The model under review builds one solid part; all positions refer to its coordinate system, in mm. A direction names the side the tool comes from. Round coordinates to 2 decimals unless told otherwise and drop trailing zeros. Write each loop counter-clockwise with the first axis right and the second up, starting at its lowest first coordinate (ties: lowest second). Pieces come first, ordered by that corner, then holes. Notation, with made-up numbers: (35, -22.5) - (58, -22.5) arc R15 ccw to (58, -6.5) - close; hole circle Ø7 at (70, -38). An arc over 180 degrees is marked (long way). Return JSON: item names as keys, results as strings.
from build123d import *

# Parameters (mm, degrees)
SKETCH1_W               = 76.2
SKETCH1_H               = 228.6
BOSS_EXTRUDE1_DEPTH     = 38.1
SKETCH2_R               = 32.512
CUT_EXTRUDE2_DEPTH      = 244.959033446
SKETCH3_W               = 5.588
SKETCH3_H               = 15.705533419
BOSS_EXTRUDE2_DEPTH     = 228.6
SKETCH4_W               = 8.89
SKETCH4_H               = 5.08
CUT_EXTRUDE3_DEPTH      = 247.899646469
CRVPATTERN1_START       = -228.6
CRVPATTERN1_OUTLINE_W   = 5.588
CRVPATTERN1_OUTLINE_H   = 5.312766709
CRVPATTERN1_DEPTH       = 228.6
CRVPATTERN1_START_2     = -165.1
CRVPATTERN1_2_OUTLINE_W = 5.588
CRVPATTERN1_2_OUTLINE_H = 5.08
CRVPATTERN1_2_DEPTH     = 101.6
CRVPATTERN1_3_OUTLINE_W = 5.588
CRVPATTERN1_3_OUTLINE_H = 5.08
CRVPATTERN1_3_DEPTH     = 54.61
CRVPATTERN1_START_3     = -54.61
CRVPATTERN1_4_OUTLINE_W = 5.588
CRVPATTERN1_4_OUTLINE_H = 5.08
CRVPATTERN1_4_DEPTH     = 54.61
CRVPATTERN1_5_OUTLINE_W = 5.588
CRVPATTERN1_5_OUTLINE_H = 5.312766709
CRVPATTERN1_5_DEPTH     = 228.6
CRVPATTERN1_6_OUTLINE_W = 5.588
CRVPATTERN1_6_OUTLINE_H = 5.08
CRVPATTERN1_6_DEPTH     = 101.6
CRVPATTERN1_7_OUTLINE_W = 5.588
CRVPATTERN1_7_OUTLINE_H = 5.08
CRVPATTERN1_7_DEPTH     = 54.61
CRVPATTERN1_8_OUTLINE_W = 5.588
CRVPATTERN1_8_OUTLINE_H = 5.08
CRVPATTERN1_8_DEPTH     = 54.61
SKETCH6_W               = 215.9
SKETCH6_H               = 53.805533419
CUT_EXTRUDE4_DEPTH      = 328.736106382
CUT_EXTRUDE5_DEPTH      = 236.189892271
BOSS_EXTRUDE4_START     = -5.588
SKETCH8_W               = 35.618239262
SKETCH8_H               = 38.1
BOSS_EXTRUDE4_DEPTH     = 5.588
SKETCH9_R               = 4.191
CUT_EXTRUDE6_DEPTH      = 236.006490398


# Read off the part's stored shape, not the designer's step: CrvPattern1
with BuildPart() as part:
    # Sketch1 → Boss-Extrude1 (new body)
    with BuildSketch(Plane(origin=(0, 0, 0), x_dir=(1, 0, 0), z_dir=(0, 1, 0))):
        with Locations((38.1, 114.3)):
            Rectangle(SKETCH1_W, SKETCH1_H)
    extrude(amount=BOSS_EXTRUDE1_DEPTH)

    # Sketch2 → Cut-Extrude2 (cut, through all)
    with BuildSketch(Plane.XY):
        with Locations((38.1, 38.1)):
            Circle(SKETCH2_R)
    extrude(amount=-CUT_EXTRUDE2_DEPTH, mode=Mode.SUBTRACT)

    # Sketch3 → Boss-Extrude2 (add)
    with BuildSketch(Plane.XY):
        with Locations((2.794, 45.95276671)):
            Rectangle(SKETCH3_W, SKETCH3_H)
        with Locations((73.406, 45.95276671)):
            Rectangle(SKETCH3_W, SKETCH3_H)
    extrude(amount=-BOSS_EXTRUDE2_DEPTH)

    # Sketch4 → Cut-Extrude3 (cut, through all)
    with BuildSketch(Plane(origin=(76.2, 0, 0), x_dir=(0, 0, -1), z_dir=(1, 0, 0))):
        with Locations((59.055, 45.95276671)):
            Rectangle(SKETCH4_W, SKETCH4_H)
        with Locations((169.545, 45.95276671)):
            Rectangle(SKETCH4_W, SKETCH4_H)
    extrude(amount=-CUT_EXTRUDE3_DEPTH, mode=Mode.SUBTRACT)


with BuildPart() as body_2:
    # CrvPattern1 outline → CrvPattern1 (new body)
    with BuildSketch(Plane.XY.offset(CRVPATTERN1_START)):
        with BuildLine():
            Line((152.4, 43.41276671), (152.4, 0))
            Line((152.4, 0), (228.6, 0))
            Line((228.6, 0), (228.6, 43.41276671))
            Line((228.6, 43.41276671), (223.012, 43.41276671))
            Line((223.012, 43.41276671), (223.012, 38.1))
            ThreePointArc((223.012, 38.1), (190.5, 5.588), (157.988, 38.1))
            Line((157.988, 38.1), (157.988, 43.41276671))
            Line((157.988, 43.41276671), (152.4, 43.41276671))
        make_face()
        with Locations((155.194, 51.149150065)):
            Rectangle(CRVPATTERN1_OUTLINE_W, CRVPATTERN1_OUTLINE_H)
        with Locations((225.806, 51.149150065)):
            Rectangle(CRVPATTERN1_OUTLINE_W, CRVPATTERN1_OUTLINE_H)
    extrude(amount=CRVPATTERN1_DEPTH)

    # CrvPattern1 2 outline → CrvPattern1 2 (add)
    with BuildSketch(Plane.XY.offset(CRVPATTERN1_START_2)):
        with Locations((155.194, 45.95276671)):
            Rectangle(CRVPATTERN1_2_OUTLINE_W, CRVPATTERN1_2_OUTLINE_H)
        with Locations((225.806, 45.95276671)):
            Rectangle(CRVPATTERN1_2_OUTLINE_W, CRVPATTERN1_2_OUTLINE_H)
    extrude(amount=CRVPATTERN1_2_DEPTH)

    # CrvPattern1 3 outline → CrvPattern1 3 (add)
    with BuildSketch(Plane.XY.offset(CRVPATTERN1_START)):
        with Locations((155.194, 45.95276671)):
            Rectangle(CRVPATTERN1_3_OUTLINE_W, CRVPATTERN1_3_OUTLINE_H)
        with Locations((225.806, 45.95276671)):
            Rectangle(CRVPATTERN1_3_OUTLINE_W, CRVPATTERN1_3_OUTLINE_H)
    extrude(amount=CRVPATTERN1_3_DEPTH)

    # CrvPattern1 4 outline → CrvPattern1 4 (add)
    with BuildSketch(Plane.XY.offset(CRVPATTERN1_START_3)):
        with Locations((155.194, 45.95276671)):
            Rectangle(CRVPATTERN1_4_OUTLINE_W, CRVPATTERN1_4_OUTLINE_H)
        with Locations((225.806, 45.95276671)):
            Rectangle(CRVPATTERN1_4_OUTLINE_W, CRVPATTERN1_4_OUTLINE_H)
    extrude(amount=CRVPATTERN1_4_DEPTH)


with BuildPart() as body_3:
    # CrvPattern1 5 outline → CrvPattern1 5 (new body)
    with BuildSketch(Plane.XY.offset(CRVPATTERN1_START)):
        with BuildLine():
            Line((76.2, 43.41276671), (76.2, 0))
            Line((76.2, 0), (152.4, 0))
            Line((152.4, 0), (152.4, 43.41276671))
            Line((152.4, 43.41276671), (146.812, 43.41276671))
            Line((146.812, 43.41276671), (146.812, 38.1))
            ThreePointArc((146.812, 38.1), (114.3, 5.588), (81.788, 38.1))
            Line((81.788, 38.1), (81.788, 43.41276671))
            Line((81.788, 43.41276671), (76.2, 43.41276671))
        make_face()
        with Locations((78.994, 51.149150065)):
            Rectangle(CRVPATTERN1_5_OUTLINE_W, CRVPATTERN1_5_OUTLINE_H)
        with Locations((149.606, 51.149150065)):
            Rectangle(CRVPATTERN1_5_OUTLINE_W, CRVPATTERN1_5_OUTLINE_H)
    extrude(amount=CRVPATTERN1_5_DEPTH)

    # CrvPattern1 6 outline → CrvPattern1 6 (add)
    with BuildSketch(Plane.XY.offset(CRVPATTERN1_START_2)):
        with Locations((78.994, 45.95276671)):
            Rectangle(CRVPATTERN1_6_OUTLINE_W, CRVPATTERN1_6_OUTLINE_H)
        with Locations((149.606, 45.95276671)):
            Rectangle(CRVPATTERN1_6_OUTLINE_W, CRVPATTERN1_6_OUTLINE_H)
    extrude(amount=CRVPATTERN1_6_DEPTH)

    # CrvPattern1 7 outline → CrvPattern1 7 (add)
    with BuildSketch(Plane.XY.offset(CRVPATTERN1_START)):
        with Locations((78.994, 45.95276671)):
            Rectangle(CRVPATTERN1_7_OUTLINE_W, CRVPATTERN1_7_OUTLINE_H)
        with Locations((149.606, 45.95276671)):
            Rectangle(CRVPATTERN1_7_OUTLINE_W, CRVPATTERN1_7_OUTLINE_H)
    extrude(amount=CRVPATTERN1_7_DEPTH)

    # CrvPattern1 8 outline → CrvPattern1 8 (add)
    with BuildSketch(Plane.XY.offset(CRVPATTERN1_START_3)):
        with Locations((78.994, 45.95276671)):
            Rectangle(CRVPATTERN1_8_OUTLINE_W, CRVPATTERN1_8_OUTLINE_H)
        with Locations((149.606, 45.95276671)):
            Rectangle(CRVPATTERN1_8_OUTLINE_W, CRVPATTERN1_8_OUTLINE_H)
    extrude(amount=CRVPATTERN1_8_DEPTH)


with BuildPart() as cut_extrude4_tool:
    # Sketch6 → Cut-Extrude4 (new, through all)
    with BuildSketch(Plane.ZY):
        with Locations((-120.65, 26.90276671)):
            Rectangle(SKETCH6_W, SKETCH6_H)
    extrude(amount=-CUT_EXTRUDE4_DEPTH)


with BuildPart() as part_1:
    add(part.part)

    # Cut-Extrude4: cut by cut_extrude4_tool
    add(cut_extrude4_tool.part, mode=Mode.SUBTRACT)


with BuildPart() as body_2_1:
    add(body_2.part)

    # Cut-Extrude4: cut by cut_extrude4_tool
    add(cut_extrude4_tool.part, mode=Mode.SUBTRACT)


with BuildPart() as body_3_1:
    add(body_3.part)

    # Cut-Extrude4: cut by cut_extrude4_tool
    add(cut_extrude4_tool.part, mode=Mode.SUBTRACT)


with BuildPart() as cut_extrude5_tool:
    # Sketch7 → Cut-Extrude5 (new, through all)
    with BuildSketch(Plane.XY):
        with BuildLine():
            Line((0, 0), (20.290880369, 0))
            ThreePointArc((20.290880369, 0), (9.524832285, 4.860053969), (0, 11.846146286))
            Line((0, 11.846146286), (0, 0))
        make_face()
        with BuildLine():
            Line((228.6, 0), (228.6, 11.846146286))
            ThreePointArc((228.6, 11.846146286), (219.075167715, 4.860053969), (208.309119631, 0))
            Line((208.309119631, 0), (228.6, 0))
        make_face()
        with BuildLine():
            Line((55.909119631, 0), (96.490880369, 0))
            ThreePointArc((96.490880369, 0), (85.724832285, 4.860053969), (76.2, 11.846146286))
            ThreePointArc((76.2, 11.846146286), (66.675167715, 4.860053969), (55.909119631, 0))
        make_face()
        with BuildLine():
            Line((132.109119631, 0), (172.690880369, 0))
            ThreePointArc((172.690880369, 0), (161.924832285, 4.860053969), (152.4, 11.846146286))
            ThreePointArc((152.4, 11.846146286), (142.875167715, 4.860053969), (132.109119631, 0))
        make_face()
    extrude(amount=-CUT_EXTRUDE5_DEPTH)


with BuildPart() as part_2:
    add(part_1.part)

    # Cut-Extrude5: cut by cut_extrude5_tool
    add(cut_extrude5_tool.part, mode=Mode.SUBTRACT)



with BuildPart() as body_2_2:
    add(body_2_1.part)

    # Cut-Extrude5: cut by cut_extrude5_tool
    add(cut_extrude5_tool.part, mode=Mode.SUBTRACT)


with BuildPart() as body_3_2:
    add(body_3_1.part)

    # Cut-Extrude5: cut by cut_extrude5_tool
    add(cut_extrude5_tool.part, mode=Mode.SUBTRACT)


with BuildPart() as part_3:
    add(part_2.part)

    add(body_2_2.part)  # Boss-Extrude4 merges body 2

    add(body_3_2.part)  # Boss-Extrude4 merges body 3
    # Sketch8 → Boss-Extrude4 (add)
    with BuildSketch(Plane(origin=(0, 0, 0), x_dir=(-1, 0, 0), z_dir=(0, -1, 0)).offset(BOSS_EXTRUDE4_START)):
        with Locations((-38.1, 6.35)):
            Rectangle(SKETCH8_W, SKETCH8_H)
        with Locations((-114.3, 6.35)):
            Rectangle(SKETCH8_W, SKETCH8_H)
        with Locations((-190.5, 6.35)):
            Rectangle(SKETCH8_W, SKETCH8_H)
    extrude(amount=BOSS_EXTRUDE4_DEPTH)

    # Sketch9 → Cut-Extrude6 (cut, through all)
    with BuildSketch(Plane(origin=(0, 5.588, 0), x_dir=(1, 0, 0), z_dir=(0, 1, 0))):
        with Locations(Location((38.1, 19.05, 0), (0, 0, 270))):
            Circle(SKETCH9_R)
        with Locations(Location((114.3, 19.05, 0), (0, 0, 270))):
            Circle(SKETCH9_R)
        with Locations(Location((190.5, 19.05, 0), (0, 0, 270))):
            Circle(SKETCH9_R)
        with Locations(Location((114.3, -6.35, 0), (0, 0, 270))):
            Circle(SKETCH9_R)
        with Locations(Location((190.5, -6.35, 0), (0, 0, 270))):
            Circle(SKETCH9_R)
        with Locations(Location((38.1, -6.35, 0), (0, 0, 270))):
            Circle(SKETCH9_R)
    extrude(amount=-CUT_EXTRUDE6_DEPTH, mode=Mode.SUBTRACT)


solid = part_3.part
(1) Add section A-A (z = 6.35). Write out the cut boundary in (x, y), plus the area to 3 significant figures.
Filled in:
{"outline": "(20.29, 0) - (33.91, 0) - (33.91, 5.59) - (20.29, 5.59) - close; (42.29, 0) - (55.91, 0) - (55.91, 5.59) - (42.29, 5.59) - close; (96.49, 0) - (110.11, 0) - (110.11, 5.59) - (96.49, 5.59) - close; (118.49, 0) - (132.11, 0) - (132.11, 5.59) - (118.49, 5.59) - close; (172.69, 0) - (186.31, 0) - (186.31, 5.59) - (172.69, 5.59) - close; (194.69, 0) - (208.31, 0) - (208.31, 5.59) - (194.69, 5.59) - close", "area": "457 mm2"}
(2) Wall thickness on line 1 (X direction, y = 1.5, z = -19.05); line 2 (Z direction, x = 190, y = 2); line 3 (X direction, y = 20, z = -0.5): over which ranges is each line inside the solid? List them lowest first.
Filled in:
{"line 1": "x = 20.29 to 33.91, 42.29 to 55.91, 96.49 to 110.11, 118.49 to 132.11, 172.69 to 186.31, 194.69 to 208.31", "line 2": "z = -25.4 to -23.21, -14.89 to 2.19, 10.51 to 12.7", "line 3": "x = 0 to 11.09, 65.11 to 87.29, 141.31 to 163.49, 217.51 to 228.6"}
(3) For faces 4 (the flat face through (5.588, 46, -6)), 5 (the cylindrical face through (85.868, 4.777, -6.261)), 6 (the flat face through (55.909, 3, 6)), 7 (the flat face through (96.491, 3, -19)), list the 3-axis set-ups (+Z, -Z, +X, -X, +Y, -Y) from which the entire face can be reached by the end or side of a thin tool; tool diameter is ignored.
Filled in:
{"face 4": "+Z, -Z, +Y", "face 5": "+Z, -Z, -Y", "face 6": "+Z, +Y, -Y", "face 7": "-Z, +Y, -Y"}
(4) Add section D-D (x = 121). Write out the cut boundary in (y, z).
Filled in:
{"outline": "(0, -25.4) - (5.59, -25.4) - (5.59, -12.7) - (6.29, -12.7) - (6.29, 0) - (5.59, 0) - (5.59, 12.7) - (0, 12.7) - close"}
(5) Add section B-B (y = 18.5). Write out the cut boundary in (x, z).
Filled in:
{"outline": "(0, -12.7) - (12.16, -12.7) - (12.16, 0) - (0, 0) - close; (64.04, -12.7) - (88.36, -12.7) - (88.36, 0) - (64.04, 0) - close; (140.24, -12.7) - (164.56, -12.7) - (164.56, 0) - (140.24, 0) - close; (216.44, -12.7) - (228.6, -12.7) - (228.6, 0) - (216.44, 0) - close"}
(6) Clearance check with flat-ended pins moving along their axes: pin 1 Ø3 at (y, z) = (1.5, -16.5) entering from +X; pin 2 Ø1 at (y, z) = (7.5, -2.5) entering from +X; pin 3 Ø1 at (y, z) = (8, -19) entering from -X; pin 4 Ø1.7 at (y, z) = (1.5, -22) entering from -X. State where each tip first meets the part, or that it passes through.
Filled in:
{"pin 1": "stops at x = 208.31", "pin 2": "stops at x = 223.88", "pin 3": "passes through", "pin 4": "stops at x = 20.29"}
(7) Add section C-C (z = -4.5). Write out the cut boundary in (x, y), plus the area to 3 significant figures.
Filled in:
{"outline": "(0, 11.85) arc R56.68 ccw to (20.29, 0) - (55.91, 0) arc R56.68 ccw to (76.2, 11.85) arc R56.68 ccw to (96.49, 0) - (132.11, 0) arc R56.68 ccw to (152.4, 11.85) arc R56.68 ccw to (172.69, 0) - (208.31, 0) arc R56.68 ccw to (228.6, 11.85) - (228.6, 53.81) - (223.01, 53.81) - (223.01, 38.1) arc R32.51 cw to (157.99, 38.1) - (157.99, 53.81) - (146.81, 53.81) - (146.81, 38.1) arc R32.51 cw to (81.79, 38.1) - (81.79, 53.81) - (70.61, 53.81) - (70.61, 38.1) arc R32.51 cw to (5.59, 38.1) - (5.59, 53.81) - (0, 53.81) - close", "area": "3,650 mm2"}
(8) Mouldability with a two-part tool opening along X and no side actions: class faces 1 (the cylindrical face through (66.818, 4.944, -6.261)), 2 (the flat face through (191, 3, 12.7)), 3 (the flat face through (0, 33, -6)) as released by +X, released by -X, zero draft, split by the parting line, or undercut.
Filled in:
{"face 1": "undercut", "face 2": "zero draft", "face 3": "released by -X"}
